from build123d import *

# Parameters (mm, degrees)
CUT_EXTRUDE1_DEPTH = 1.3


with BuildPart() as part:
    # Sketch1 → Revolve1 (revolve)
    with BuildSketch(Plane(origin=(0, 0, 0), x_dir=(0, 0, -1), z_dir=(1, 0, 0))):
        with BuildLine():
            Line((0, 0), (0, 2.45))
            Line((0, 2.45), (0.3, 2.75))
            Line((0.3, 2.75), (2.785, 2.75))
            Line((2.785, 2.75), (3, 2.535))
            Line((3, 2.535), (3, 1.8))
            ThreePointArc((3, 1.8), (3.015193643, 1.74701055), (3.056157637, 1.710123155))
            Line((3.056157637, 1.710123155), (3.466157637, 1.510123155))
            ThreePointArc((3.466157637, 1.510123155), (3.48750205, 1.50256365), (3.51, 1.5))
            Line((3.51, 1.5), (8.75, 1.5))
            Line((8.75, 1.5), (9, 1.25))
            Line((9, 1.25), (9, 0))
            Line((9, 0), (0, 0))
        make_face()
    revolve(axis=Axis((0, 0, 0), (0, 0, -1)))

    # Sketch2 → Cut-Extrude1 (cut)
    with BuildSketch(Plane.XY):
        Polygon((0, 1.443375673), (-1.25, 0.721687836), (-1.25, -0.721687836), (0, -1.443375673), (1.25, -0.721687836), (1.25, 0.721687836), align=None)
    extrude(amount=-CUT_EXTRUDE1_DEPTH, mode=Mode.SUBTRACT)

    # Sketch3 → Cut-Revolve2 (revolve, cut)
    with BuildSketch(Plane(origin=(0, 0, 0), x_dir=(0, 0, -1), z_dir=(1, 0, 0))):
        Polygon((1.3, 0), (1.3, 1.25), (2.021687836, 0), align=None)
    revolve(axis=Axis((0, 0, -1.3), (0, 0, -1)), mode=Mode.SUBTRACT)

    # Sketch4 → Cut-Revolve3 (revolve, cut)
    with BuildSketch(Plane(origin=(0, 0, 0), x_dir=(0, 0, -1), z_dir=(1, 0, 0))):
        Polygon((0, 1.443375673), (0, 1.25), (0.051814855, 1.25), align=None)
    revolve(axis=Axis((0, 0, 0), (0, 0, -1)), mode=Mode.SUBTRACT)


solid = part.part
Geometry: final body of the model. Coordinates: model frame, mm. A direction names the side the tool comes from. Round coordinates to 2 decimals unless told otherwise and drop trailing zeros. Order: outer loops, then holes, each group sorted by start corner. A loop starts at its lowest first (then second) coordinate and runs counter-clockwise, first axis right, second up. Notation, with made-up numbers: (-11.5, 87.5) -> (30.5, 87.5) arc R16 ccw to (30.5, 102.5) -> close; hole circle Ø4 at (80.25, -38.5). An arc over 180 degrees is marked (long way). Put each result on its own line as item: value. Start each with the question number.
Q1. Section B-B on z = -1.75. Return the cut outline in (x, y).
Q2. First-contact query: pin 1 (0.7 mm diameter, centred on y = 0.5, z = -1, fed in from +X); pin 2 (2 mm diameter, centred on y = -2, z = -7, fed in from +X). Flat tips, straight axial feed; report the tip coordinate or a pass-through.
Q3. Pull-direction query (X, two-part tool) for faces 1 (the cylindrical face through (-2.685, -0.596, -1.56)), 2 (the flat face through (0, 0, -9)), 3 (the flat face through (0.616, -1.088, -0.641)); classes: +X half, -X half, draft (parallel to the pull), parting line (faces both ways), or undercut.
Q4. Reachability of faces 4 (the flat face through (1.25, 0, -1)), 5 (the flat face through (-2, 0, 0)), 6 (the flat face through (-1, -2, -3)) from +Z, -Z, +X, -X, +Y, -Y: full face, straight path, thin tool, end or side. Return the list, or none.
Q5. Section A-A on z = -4.5. Return the cut outline in (x, y), and give its area (3 significant figures).
Q6. Line query: probe 1 along Z at (x, y) = (1.7, -1.6); probe 2 along X at (y, z) = (0.7, -1); probe 3 along X at (y, z) = (-1, -5.5). Output: solid intervals per line, ascending.
Ans:
1. outline: circle Ø5.5 at (0, 0); hole circle Ø0.94 at (0, 0)
2. pin 1: stops at x = 2.75
2. pin 2: stops at x = 1.12
3. face 1: parting line
3. face 2: draft
3. face 3: undercut
4. face 4: +Z
4. face 5: +Z, +X, -X, +Y, -Y
4. face 6: -Z
5. outline: circle Ø3 at (0, 0)
5. area: 7.07 mm2
6. probe 1: z = -3 to 0
6. probe 2: x = -2.66 to -1.25, 1.25 to 2.66
6. probe 3: x = -1.12 to 1.12
